from build123d import *

# Parameters (mm, degrees)
SKETCH_1_W               = 380
SKETCH_1_H               = 200
EXTRUDE_1_DEPTH          = 12
SKETCH_2_R               = 13
CUT_EXTRUDE_1_DEPTH      = 430.585847067
MIRROR_2_COPY_1_SKETCH_R = 13
MIRROR_2_COPY_1_DEPTH    = 430.585847067


with BuildPart() as part:
    # 草图1 → 凸台-拉伸1 (new body)
    with BuildSketch(Plane.XY):
        with Locations((190, 100)):
            Rectangle(SKETCH_1_W, SKETCH_1_H)
    extrude(amount=EXTRUDE_1_DEPTH)

    # 草图2 → 切除-拉伸1 (cut, through all)
    with BuildSketch(Plane.XY.offset(12)):
        with Locations((41.004801127, 41.686787837)):
            Circle(SKETCH_2_R)
    cut_extrude_1 = extrude(amount=-CUT_EXTRUDE_1_DEPTH, mode=Mode.SUBTRACT)

    # 镜向1: 切除-拉伸1 across plane
    add(cut_extrude_1.mirror(Plane.ZX.offset(100)), mode=Mode.SUBTRACT)

    # 镜向2: 切除-拉伸1 across plane
    add(cut_extrude_1.mirror(Plane(origin=(190, 0, 0), x_dir=(0, 0, 1), z_dir=(1, 0, 0))), mode=Mode.SUBTRACT)

    # 镜向2 copy 1 sketch → 镜向2 copy 1 (cut, through all)
    with BuildSketch(Plane(origin=(380, 200, 12), x_dir=(-1, 0, 0), z_dir=(0, 0, 1))):
        with Locations((41.004801127, 41.686787837)):
            Circle(MIRROR_2_COPY_1_SKETCH_R)
    extrude(amount=-MIRROR_2_COPY_1_DEPTH, mode=Mode.SUBTRACT)


solid = part.part
For this review, take the finished solid that the model builds, in its own axes (mm). Round coordinates to 2 decimals unless told otherwise and drop trailing zeros. Write each loop counter-clockwise with the first axis right and the second up, starting at its lowest first coordinate (ties: lowest second). Pieces come first, ordered by that corner, then holes. Notation, with made-up numbers: (52.5, -35) - (111.5, -35) arc R15 ccw to (111.5, -31) - close; hole circle Ø10 at (12.5, 23.25). An arc over 180 degrees is marked (long way). Use a Markdown table: item, result.
Q1. The part is to be moulded in two halves that separate along Y. For faces 1 (the cylindrical face through (39.312, 54.576, 6.084)), 2 (the flat face through (187, 0, 6)), 3 (the cylindrical face through (326.6, 45.6, 6.1)), 4 (the flat face through (187, 200, 6)), say which applies: pulls with the +Y half, pulls with the -Y half, needs draft (parallel to the pull), parting line crosses it, or undercut.
Derived:
| item | result |
|---|---|
| face 1 | undercut |
| face 2 | pulls with the -Y half |
| face 3 | undercut |
| face 4 | pulls with the +Y half |
Q2. We need section A-A (y = 50.5). Give the boundary of the cut face in (x, z).
Derived:
| item | result |
|---|---|
| outline | (0, 0) - (31.45, 0) - (31.45, 12) - (0, 12) - close; (50.56, 0) - (329.44, 0) - (329.44, 12) - (50.56, 12) - close; (348.55, 0) - (380, 0) - (380, 12) - (348.55, 12) - close |
Q3. We need section C-C (z = 7.75). Give the boundary of the cut face in (x, y), plus the area to 3 significant figures.
Derived:
| item | result |
|---|---|
| outline | (0, 0) - (380, 0) - (380, 200) - (0, 200) - close; hole circle Ø26 at (41, 41.69); hole circle Ø26 at (41, 158.31); hole circle Ø26 at (339, 41.69); hole circle Ø26 at (339, 158.31) |
| area | 73,900 mm2 |
Q4. Wall thickness on line 1 along X through (y, z) = (149.5, 7.5); line 2 along X through (y, z) = (154.5, 7.25): over which ranges is each line inside the solid? List them lowest first.
Derived:
| item | result |
|---|---|
| line 1 | x = 0 to 31.45, 50.56 to 329.44, 348.55 to 380 |
| line 2 | x = 0 to 28.58, 53.43 to 326.57, 351.42 to 380 |
Q5. Clearance check with a flat-ended pin moving along its axis: pin 1 (15.5 mm diameter, centred on x = 41, y = 158.31, fed in from -Z). State where the tip first meets the part, or that it passes through.
Derived:
| item | result |
|---|---|
| pin 1 | passes through |
Q6. We need section B-B (x = 345). Give the boundary of the cut face in (y, z).
Derived:
| item | result |
|---|---|
| outline | (0, 0) - (30.16, 0) - (30.16, 12) - (0, 12) - close; (53.22, 0) - (146.78, 0) - (146.78, 12) - (53.22, 12) - close; (169.84, 0) - (200, 0) - (200, 12) - (169.84, 12) - close |
